```python
from build123d import *

# Parameters (mm, degrees)
EXTRUDE2_DEPTH      = 6.35
SKETCH3_OUTSIDE_W   = 18.322
SKETCH3_OUTSIDE_H   = 16.747
CUT_EXTRUDE1_DEPTH  = 7.62
SKETCH4_W           = 6.6294
SKETCH4_H           = 5.959117839
CUT_EXTRUDE2_DEPTH  = 12.7
EXTRUDE3_DEPTH      = 2.54
EXTRUDE3_DEPTH_BACK = 3.5052
SKETCH5_W           = 0.7112
SKETCH5_H           = 0.3048
SKETCH6_R           = 1.7526
EXTRUDE4_DEPTH      = 5.3


with BuildPart() as part:
    # Sketch2 → Extrude2 (new, symmetric)
    with BuildSketch(Plane(origin=(0, 0, 0), x_dir=(0, 0, -1), z_dir=(1, 0, 0))):
        Polygon((0, 0), (5.0292, 0), (5.0292, -3.5052), (5.7404, -3.5052), (5.7404, 0), (6.5532, 0), (6.5532, 2.025013386), (4.5212, 2.025013386), (4.5212, 5.588), (3.556, 5.588), (3.556, 7.62), (0, 7.62), align=None)
    extrude(amount=EXTRUDE2_DEPTH, both=True)

    # Sketch3 outside → Cut-Extrude1 (cut, symmetric)
    with BuildSketch(Plane.XY):
        with Locations((0, 2.0575)):
            Rectangle(SKETCH3_OUTSIDE_W, SKETCH3_OUTSIDE_H)
        with BuildLine():
            Line((-3.3147, 0.6858), (3.3147, 0.6858))
            Line((3.3147, 0.6858), (3.3147, -0.396973009))
            Line((3.3147, -0.396973009), (3.748326519, -1.588352079))
            Line((3.748326519, -1.588352079), (2.978268534, -3.704069007))
            Line((2.978268534, -3.704069007), (3.3147, -3.826520046))
            Line((3.3147, -3.826520046), (4.129326519, -1.588352079))
            Line((4.129326519, -1.588352079), (3.6957, -0.396973009))
            Line((3.6957, -0.396973009), (3.6957, 5.588))
            Line((3.6957, 5.588), (3.3147, 5.588))
            Line((3.3147, 5.588), (3.3147, 6.7818))
            ThreePointArc((3.3147, 6.7818), (3.165910245, 7.141010245), (2.8067, 7.2898))
            Line((2.8067, 7.2898), (-2.8067, 7.2898))
            ThreePointArc((-2.8067, 7.2898), (-3.165910245, 7.141010245), (-3.3147, 6.7818))
            Line((-3.3147, 6.7818), (-3.3147, 5.588))
            Line((-3.3147, 5.588), (-3.6957, 5.588))
            Line((-3.6957, 5.588), (-3.6957, -0.396973009))
            Line((-3.6957, -0.396973009), (-4.129326519, -1.588352079))
            Line((-4.129326519, -1.588352079), (-3.3147, -3.826520046))
            Line((-3.3147, -3.826520046), (-2.978268534, -3.704069007))
            Line((-2.978268534, -3.704069007), (-3.748326519, -1.588352079))
            Line((-3.748326519, -1.588352079), (-3.3147, -0.396973009))
            Line((-3.3147, -0.396973009), (-3.3147, 0.6858))
        make_face(mode=Mode.SUBTRACT)
    extrude(amount=CUT_EXTRUDE1_DEPTH, both=True, mode=Mode.SUBTRACT)

    # Sketch4 → Cut-Extrude2 (cut)
    with BuildSketch(Plane(origin=(0, 0, 0), x_dir=(1, 0, 0), z_dir=(0, 1, 0))):
        with Locations((0, 6.535558919)):
            Rectangle(SKETCH4_W, SKETCH4_H)
    extrude(amount=CUT_EXTRUDE2_DEPTH, mode=Mode.SUBTRACT)

    # Sketch5 → Extrude3 (add, two sides: drawn at the far end of the back side and taken through both)
    with BuildSketch(Plane(origin=(0, 0, 0), x_dir=(1, 0, 0), z_dir=(0, 1, 0)).offset(-EXTRUDE3_DEPTH_BACK)):
        with Locations((2.2479, 2.54)):
            Rectangle(SKETCH5_W, SKETCH5_H)
        with Locations((-2.2479, 2.54)):
            Rectangle(SKETCH5_W, SKETCH5_H)
    extrude(amount=EXTRUDE3_DEPTH + EXTRUDE3_DEPTH_BACK)

    # Sketch6 → Extrude4 (add)
    with BuildSketch(Plane.XY):
        with Locations(Location((0, 3.9878, 0), (0, 0, 180))):
            Circle(SKETCH6_R)
    extrude(amount=EXTRUDE4_DEPTH)


solid = part.part
```
CAD build for the part. Positions are in the model's coordinates, mm. A direction names the side the tool comes from. Round coordinates to 2 decimals unless told otherwise and drop trailing zeros. Order: outer loops, then holes, each group sorted by start corner. A loop starts at its lowest first (then second) coordinate and runs counter-clockwise, first axis right, second up.
Item 1: Tool access for faces 4 (the face through (-0.81, 5.54, 2.61)), 5 (the face through (-3.315, 2, -4)), 6 (the face through (-3.9, -1.7, -5.029)), 7 (the face through (3.8, -1.9, -5.74)): list every direction of +Z, -Z, +X, -X, +Y, -Y with a clear straight run to the whole face (end or side of a thin tool).
Item 2: Saw through at C-C on y = 6.25. Write the cut outline in (x, z), then the cut area to 3 significant figures.
Item 3: Mould opens along X. For faces 1 (the face through (-3.8, -1.9, -5.74)), 2 (the face through (3.315, 6, -2)), 3 (the face through (0, 4, -3.556)) say: pulls with the +X half, pulls with the -X half, needs draft (parallel to the pull), parting line crosses it, or undercut.
Item 4: Pin check, flat tips, straight feed: pin 1 (2 mm diameter, centred on x = -1, y = 4, fed in from -Z); pin 2 (0.6 mm diameter, centred on x = -2, y = -1.5, fed in from -Z); pin 3 (1.5 mm diameter, centred on x = -2.5, y = 2.5, fed in from +Z). Stop position of each tip, or through.
Item 5: Probe line 1 along Z through (x, y) = (3.25, 6.5); line 2 along X through (y, z) = (6.75, -2.75); line 3 along Y through (x, z) = (-1.5, -1.5). List the from-to ranges inside material, lowest first.
Item 6: Saw through at D-D on x = -1. Write the cut outline in (y, z), then the cut area to 3 significant figures.
Item 7: Saw through at A-A on z = -5.25. Write the cut outline in (x, y), then the cut area to 3 significant figures.
Item 8: Saw through at B-B on x = 0. Write the cut outline in (y, z), then the cut area to 3 significant figures.
Reported:
1. face 4: +Z
1. face 5: -Z
1. face 6: +Z, +X, -X, -Y
1. face 7: -Z, +X, -X, -Y
2. outline: (-3.31, -3.56) - (3.31, -3.56) - (3.31, 0) - (-3.31, 0) - close
2. area: 23.6 mm2
3. face 1: needs draft
3. face 2: pulls with the +X half
3. face 3: undercut
4. pin 1: stops at z = -3.56
4. pin 2: stops at z = -2.69
4. pin 3: stops at z = 0
5. line 1: z = -3.56 to 0
5. line 2: x = -3.31 to 3.31
5. line 3: y = 0.69 to 7.29
6. outline: (0.69, -3.56) - (7.29, -3.56) - (7.29, 0) - (5.43, 0) - (5.43, 5.3) - (2.55, 5.3) - (2.55, 0) - (0.69, 0) - close
6. area: 38.7 mm2
7. outline: (-4.13, -1.59) - (-3.43, -3.51) - (-3.05, -3.51) - (-3.75, -1.59) - (-3.31, -0.4) - (-3.31, 2.03) - (-3.7, 2.03) - (-3.7, -0.4) - close; (3.05, -3.51) - (3.43, -3.51) - (4.13, -1.59) - (3.7, -0.4) - (3.7, 2.03) - (3.31, 2.03) - (3.31, -0.4) - (3.75, -1.59) - close
7. area: 4.21 mm2
8. outline: (0.69, -3.56) - (7.29, -3.56) - (7.29, 0) - (5.74, 0) - (5.74, 5.3) - (2.24, 5.3) - (2.24, 0) - (0.69, 0) - close
8. area: 42.1 mm2
